```python
from build123d import *

# Parameters (mm, degrees)
F0_R     = 11.25
F1_DEPTH = 7.62
F2_R     = 2.54


with BuildPart() as f1:
    # F0 (on Top) → F1 (new body)
    with BuildSketch(Plane.XY):
        with BuildLine():
            ThreePointArc((13.695194, -2.757274), (13.901129, -1.385467), (13.97, 0))
            ThreePointArc((13.97, 0), (12.456401, 6.324474), (8.243591, 11.27848))
            ThreePointArc((8.243591, 11.27848), (-5.057937, 13.022218), (-13.695194, 2.757274))
            ThreePointArc((-13.695194, 2.757274), (-13.022218, -5.057937), (-8.243591, -11.27848))
            ThreePointArc((-8.243591, -11.27848), (5.057937, -13.022218), (13.695194, -2.757274))
        make_face()
        Circle(F0_R, mode=Mode.SUBTRACT)
        with BuildLine():
            ThreePointArc((8.243591, 11.27848), (12.456401, 6.324474), (13.97, 0))
            ThreePointArc((13.97, 0), (13.901129, -1.385467), (13.695194, -2.757274))
            Line((13.695194, -2.757274), (18.046504, -3.400007))
            Line((18.046504, -3.400007), (20.647889, -3.784257))
            Line((20.647889, -3.784257), (23.234406, -4.166312))
            Line((23.234406, -4.166312), (26.258385, -4.612984))
            Line((26.258385, -4.612984), (28.523248, -4.947527))
            Line((28.523248, -4.947527), (30.968487, -5.308713))
            Line((30.968487, -5.308713), (32.656681, -5.558076))
            Line((32.656681, -5.558076), (35.562277, -5.987262))
            Line((35.562277, -5.987262), (37.618638, -6.291007))
            Line((37.618638, -6.291007), (40.230147, -6.676753))
            Line((40.230147, -6.676753), (42.585731, -7.024697))
            Line((42.585731, -7.024697), (44.640029, -7.328137))
            Line((44.640029, -7.328137), (46.360764, -7.582307))
            Line((46.360764, -7.582307), (45.977047, -6.092634))
            Line((45.977047, -6.092634), (45.382247, -3.783485))
            Line((45.382247, -3.783485), (44.2688, 0.539161))
            Line((44.2688, 0.539161), (43.710486, 2.706662))
            Line((43.710486, 2.706662), (43.192849, 4.716242))
            Line((43.192849, 4.716242), (39.974761, 5.320486))
            Line((39.974761, 5.320486), (37.129923, 5.854646))
            Line((37.129923, 5.854646), (34.206946, 6.403478))
            Line((34.206946, 6.403478), (31.410099, 6.928627))
            Line((31.410099, 6.928627), (28.772873, 7.423805))
            Line((28.772873, 7.423805), (26.212834, 7.90449))
            Line((26.212834, 7.90449), (23.747829, 8.367331))
            Line((23.747829, 8.367331), (21.698637, 8.752097))
            Line((21.698637, 8.752097), (19.441536, 9.175901))
            Line((19.441536, 9.175901), (17.487376, 9.542823))
            Line((17.487376, 9.542823), (15.022369, 10.005664))
            Line((15.022369, 10.005664), (13.060459, 10.374042))
            Line((13.060459, 10.374042), (11.307054, 10.70327))
            Line((11.307054, 10.70327), (9.495402, 11.043434))
            Line((9.495402, 11.043434), (8.243591, 11.27848))
        make_face()
        with BuildLine():
            ThreePointArc((-8.243591, -11.27848), (-13.022218, -5.057937), (-13.695194, 2.757274))
            Line((-13.695194, 2.757274), (-18.046504, 3.400007))
            Line((-18.046504, 3.400007), (-20.647889, 3.784257))
            Line((-20.647889, 3.784257), (-23.234406, 4.166312))
            Line((-23.234406, 4.166312), (-26.258385, 4.612984))
            Line((-26.258385, 4.612984), (-28.523248, 4.947527))
            Line((-28.523248, 4.947527), (-30.968487, 5.308713))
            Line((-30.968487, 5.308713), (-32.656681, 5.558076))
            Line((-32.656681, 5.558076), (-35.562277, 5.987262))
            Line((-35.562277, 5.987262), (-37.618638, 6.291007))
            Line((-37.618638, 6.291007), (-40.230147, 6.676753))
            Line((-40.230147, 6.676753), (-42.585731, 7.024697))
            Line((-42.585731, 7.024697), (-44.640029, 7.328137))
            Line((-44.640029, 7.328137), (-46.360764, 7.582307))
            Line((-46.360764, 7.582307), (-45.977047, 6.092634))
            Line((-45.977047, 6.092634), (-45.382247, 3.783485))
            Line((-45.382247, 3.783485), (-44.2688, -0.539161))
            Line((-44.2688, -0.539161), (-43.710486, -2.706662))
            Line((-43.710486, -2.706662), (-43.192849, -4.716242))
            Line((-43.192849, -4.716242), (-39.974761, -5.320486))
            Line((-39.974761, -5.320486), (-37.129923, -5.854646))
            Line((-37.129923, -5.854646), (-34.206946, -6.403478))
            Line((-34.206946, -6.403478), (-31.410099, -6.928627))
            Line((-31.410099, -6.928627), (-28.772873, -7.423805))
            Line((-28.772873, -7.423805), (-26.212834, -7.90449))
            Line((-26.212834, -7.90449), (-23.747829, -8.367331))
            Line((-23.747829, -8.367331), (-21.698637, -8.752097))
            Line((-21.698637, -8.752097), (-19.441536, -9.175901))
            Line((-19.441536, -9.175901), (-17.487376, -9.542823))
            Line((-17.487376, -9.542823), (-15.022369, -10.005664))
            Line((-15.022369, -10.005664), (-13.060459, -10.374042))
            Line((-13.060459, -10.374042), (-11.307054, -10.70327))
            Line((-11.307054, -10.70327), (-9.495402, -11.043434))
            Line((-9.495402, -11.043434), (-8.243591, -11.27848))
        make_face()
        Polygon((10.707353, 12.637032), (9.495402, 11.043434), (11.307054, 10.70327), align=None)
        Polygon((12.871755, 12.391077), (11.307054, 10.70327), (13.060459, 10.374042), align=None)
        Polygon((14.64263, 11.948359), (13.060459, 10.374042), (15.022369, 10.005664), align=None)
        Polygon((16.610269, 11.948359), (15.022369, 10.005664), (17.487376, 9.542823), align=None)
        Polygon((19.020624, 11.27848), (17.487376, 9.542823), (19.441536, 9.175901), align=None)
        Polygon((21.135837, 11.27848), (19.441536, 9.175901), (21.698637, 8.752097), align=None)
        Polygon((23.239078, 11.27848), (21.698637, 8.752097), (23.747829, 8.367331), align=None)
        Polygon((25.566199, 10.789929), (23.747829, 8.367331), (26.212834, 7.90449), align=None)
        Polygon((28.202849, 10.374042), (26.212834, 7.90449), (28.772873, 7.423805), align=None)
        Polygon((30.480421, 9.542823), (28.772873, 7.423805), (31.410099, 6.928627), align=None)
        Polygon((33.220999, 9.175901), (31.410099, 6.928627), (34.206946, 6.403478), align=None)
        Polygon((36.099512, 8.752097), (34.206946, 6.403478), (37.129923, 5.854646), align=None)
        Polygon((38.971896, 8.140481), (37.129923, 5.854646), (39.974761, 5.320486), align=None)
        Polygon((41.253339, 7.882453), (39.974761, 5.320486), (43.192849, 4.716242), align=None)
        Polygon((46.070598, 4.716242), (43.192849, 4.716242), (43.710486, 2.706662), align=None)
        Polygon((46.741366, 2.13757), (43.710486, 2.706662), (44.2688, 0.539161), align=None)
        Polygon((44.2688, 0.539161), (45.382247, -3.783485), (47.609445, -2.1535), (44.776806, -1.055378), (47.007285, -0.480841), align=None)
        Polygon((45.382247, -3.783485), (45.977047, -6.092634), (48.144694, -4.294504), align=None)
        Polygon((45.977047, -6.092634), (46.360764, -7.582307), (48.332162, -6.857038), align=None)
        Polygon((46.360764, -7.582307), (44.640029, -7.328137), (45.839909, -9.274097), align=None)
        Polygon((44.640029, -7.328137), (42.585731, -7.024697), (43.723498, -9.274097), align=None)
        Polygon((42.585731, -7.024697), (40.230147, -6.676753), (41.177191, -9.274097), align=None)
        Polygon((40.230147, -6.676753), (37.618638, -6.291007), (38.597815, -8.976477), align=None)
        Polygon((37.618638, -6.291007), (35.562277, -5.987262), (35.883938, -8.254709), align=None)
        Polygon((35.562277, -5.987262), (32.656681, -5.558076), (33.505198, -7.885202), align=None)
        Polygon((32.656681, -5.558076), (30.968487, -5.308713), (31.554129, -7.582307), align=None)
        Polygon((30.968487, -5.308713), (28.523248, -4.947527), (29.330876, -7.162509), align=None)
        Polygon((28.523248, -4.947527), (26.258385, -4.612984), (26.836419, -6.857038), align=None)
        Polygon((26.258385, -4.612984), (23.234406, -4.166312), (24.006179, -7.162509), align=None)
        Polygon((23.234406, -4.166312), (20.647889, -3.784257), (21.518074, -7.162509), align=None)
        Polygon((20.647889, -3.784257), (18.046504, -3.400007), (19.015666, -7.162509), align=None)
        Polygon((18.046504, -3.400007), (13.695194, -2.757274), (16.351812, -7.162509), align=None)
        Polygon((-10.707353, -12.637032), (-9.495402, -11.043434), (-11.307054, -10.70327), align=None)
        Polygon((-12.871755, -12.391077), (-11.307054, -10.70327), (-13.060459, -10.374042), align=None)
        Polygon((-14.64263, -11.948359), (-13.060459, -10.374042), (-15.022369, -10.005664), align=None)
        Polygon((-16.610269, -11.948359), (-15.022369, -10.005664), (-17.487376, -9.542823), align=None)
        Polygon((-19.020624, -11.27848), (-17.487376, -9.542823), (-19.441536, -9.175901), align=None)
        Polygon((-21.135837, -11.27848), (-19.441536, -9.175901), (-21.698637, -8.752097), align=None)
        Polygon((-23.239078, -11.27848), (-21.698637, -8.752097), (-23.747829, -8.367331), align=None)
        Polygon((-25.566199, -10.789929), (-23.747829, -8.367331), (-26.212834, -7.90449), align=None)
        Polygon((-28.202849, -10.374042), (-26.212834, -7.90449), (-28.772873, -7.423805), align=None)
        Polygon((-33.220999, -9.175901), (-31.410099, -6.928627), (-34.206946, -6.403478), align=None)
        Polygon((-38.971896, -8.140481), (-37.129923, -5.854646), (-39.974761, -5.320486), align=None)
        Polygon((-41.253339, -7.882453), (-39.974761, -5.320486), (-43.192849, -4.716242), align=None)
        Polygon((-30.480421, -9.542823), (-28.772873, -7.423805), (-31.410099, -6.928627), align=None)
        Polygon((-36.099512, -8.752097), (-34.206946, -6.403478), (-37.129923, -5.854646), align=None)
        Polygon((-46.070598, -4.716242), (-43.192849, -4.716242), (-43.710486, -2.706662), align=None)
        Polygon((-43.710486, -2.706662), (-44.2688, -0.539161), (-46.741366, -2.13757), align=None)
        Polygon((-45.382247, 3.783485), (-45.977047, 6.092634), (-48.144694, 4.294504), align=None)
        Polygon((-45.977047, 6.092634), (-46.360764, 7.582307), (-48.332162, 6.857038), align=None)
        Polygon((-46.360764, 7.582307), (-44.640029, 7.328137), (-45.839909, 9.274097), align=None)
        Polygon((-44.640029, 7.328137), (-42.585731, 7.024697), (-43.723498, 9.274097), align=None)
        Polygon((-42.585731, 7.024697), (-40.230147, 6.676753), (-41.177191, 9.274097), align=None)
        Polygon((-40.230147, 6.676753), (-37.618638, 6.291007), (-38.597815, 8.976477), align=None)
        Polygon((-37.618638, 6.291007), (-35.562277, 5.987262), (-35.883938, 8.254709), align=None)
        Polygon((-32.656681, 5.558076), (-30.968487, 5.308713), (-31.554129, 7.582307), align=None)
        Polygon((-30.968487, 5.308713), (-28.523248, 4.947527), (-29.330876, 7.162509), align=None)
        Polygon((-28.523248, 4.947527), (-26.258385, 4.612984), (-26.836419, 6.857038), align=None)
        Polygon((-44.2688, -0.539161), (-45.382247, 3.783485), (-47.609445, 2.1535), (-44.776806, 1.055378), (-47.007285, 0.480841), align=None)
        Polygon((-35.562277, 5.987262), (-32.656681, 5.558076), (-33.505198, 7.885202), align=None)
        Polygon((-26.258385, 4.612984), (-23.234406, 4.166312), (-24.006179, 7.162509), align=None)
        Polygon((-23.234406, 4.166312), (-20.647889, 3.784257), (-21.518074, 7.162509), align=None)
        Polygon((-20.647889, 3.784257), (-18.046504, 3.400007), (-19.015666, 7.162509), align=None)
        Polygon((-18.046504, 3.400007), (-13.695194, 2.757274), (-16.351812, 7.162509), align=None)
    extrude(amount=F1_DEPTH)

    # F2
    f2_edges = [f1.edges().sort_by_distance(p)[0] for p in [
        (-46.360764, 7.582307, 3.81),
        (-43.192849, -4.716242, 3.81),
        (46.360764, -7.582307, 3.81),
        (43.192849, 4.716242, 3.81),
    ]]
    fillet(f2_edges, radius=F2_R)


solid = f1.part
```
Verification items for the finished model (mm, model axes). Coordinates: 2 decimals unless noted, no trailing zeros. Loops run counter-clockwise (first coordinate to the right, second up) from the corner with the lowest first, then second, coordinate; pieces in that order, holes last. Notation, with made-up numbers: (61.5, 14.5) - (112.5, 14.5) arc R8 ccw to (112.5, 20.5) - close; hole circle Ø8 at (82, 66). An arc over 180 degrees is marked (long way). Return JSON: item names as keys, results as strings.
1. Section check A-A, the plane x = 0. Record the boundary of the cut face in (y, z).
Established:
{"outline": "(-13.97, 0) - (-11.25, 0) - (-11.25, 7.62) - (-13.97, 7.62) - close; (11.25, 0) - (13.97, 0) - (13.97, 7.62) - (11.25, 7.62) - close"}
2. Go/stop test with flat-tipped pins: pin 1 (3 mm diameter, centred on x = -14.5, z = 4.5, fed in from -Y); pin 2 (1.2 mm diameter, centred on x = 45.5, z = 2.5, fed in from +Y); pin 3 (1.6 mm diameter, centred on x = -45.5, z = 4.5, fed in from -Y). Record where each tip stops, or that it passes through.
Established:
{"pin 1": "stops at y = -11.95", "pin 2": "stops at y = 4.72", "pin 3": "stops at y = -4.72"}
3. Thickness scan on L1, parallel to Y at x = 0, z = 2.5; L2, parallel to Y at x = -10, z = 5. Record the ranges inside material, lowest first.
Established:
{"L1": "y = -13.97 to -11.25, 11.25 to 13.97", "L2": "y = -11.71 to -5.15, 5.15 to 9.76"}
4. Mould release check, pull along Y, two halves, no side actions. Record for faces 1 (the cylindrical face through (-43.39, -5.03, 3.86)), 2 (the flat face through (47.17, -6.48, 3.76)), 3 (the flat face through (-11.4, 0.2, 7.62)): +Y half, -Y half, draft (parallel to the pull), parting line (faces both ways), or undercut.
Established:
{"face 1": "-Y half", "face 2": "undercut", "face 3": "draft"}
